```python
from build123d import *

# Parameters (mm, degrees)
SKETCH1_W                    = 44.45
SKETCH1_H                    = 12.7
SKETCH1_H_2                  = 15.875
SKETCH1_W_2                  = 41.275
BOSS_EXTRUDE1_DEPTH          = 3.175
SKETCH3_R                    = 14.2875
CUT_EXTRUDE1_DEPTH           = 68.351920908
F_18_0_1695_DIAMETER_HOLE1_D = 4.3053
CIRPATTERN1_COUNT            = 4
FILLET1_R                    = 6.35
FILLET2_R                    = 6.35
F_18_0_1695_DIAMETER_HOLE2_D = 4.3053


with BuildPart() as part:
    # Sketch1 → Boss-Extrude1 (new body)
    with BuildSketch(Plane(origin=(0, 0, 0), x_dir=(1, 0, 0), z_dir=(0, 1, 0))):
        Rectangle(SKETCH1_W, SKETCH1_H)
        with Locations((0, -14.2875)):
            Rectangle(SKETCH1_W, SKETCH1_H_2)
        with Locations((42.8625, 0)):
            Rectangle(SKETCH1_W_2, SKETCH1_H)
        with Locations((0, 14.2875)):
            Rectangle(SKETCH1_W, SKETCH1_H_2)
        with Locations((-42.8625, 0)):
            Rectangle(SKETCH1_W_2, SKETCH1_H)
    extrude(amount=BOSS_EXTRUDE1_DEPTH)

    # Sketch3 → Cut-Extrude1 (cut, through all)
    with BuildSketch(Plane(origin=(0, 3.175, 0), x_dir=(1, 0, 0), z_dir=(0, 1, 0))):
        with Locations(Location((0, 0, 0), (0, 0, 270))):
            Circle(SKETCH3_R)
    extrude(amount=-CUT_EXTRUDE1_DEPTH, mode=Mode.SUBTRACT)

    # #18 (0.1695) Diameter Hole1 (through all)
    with Locations(Plane(origin=(0, 3.175, 0), x_dir=(1, 0, 0), z_dir=(0, 1, 0))):
        with Locations((-15.715448212, -15.715448212)):
            f_18_0_1695_diameter_hole1 = Hole(F_18_0_1695_DIAMETER_HOLE1_D / 2)

    # CirPattern1: #18 (0.1695) Diameter Hole1 ×4 about axis
    cirpattern1_axis = Axis((0, 0, 0), (0, 1, 0))
    for i in range(1, CIRPATTERN1_COUNT):
        add(f_18_0_1695_diameter_hole1.rotate(cirpattern1_axis, i * 360 / CIRPATTERN1_COUNT), mode=Mode.SUBTRACT)

    # Fillet1
    fillet1_edges = [part.edges().sort_by_distance(p)[0] for p in [
        (-22.225, 1.5875, 6.35),
        (-22.225, 1.5875, -6.35),
        (22.225, 1.5875, -6.35),
        (22.225, 1.5875, 6.35),
    ]]
    fillet(fillet1_edges, radius=FILLET1_R)

    # Fillet2
    fillet2_edges = [part.edges().sort_by_distance(p)[0] for p in [
        (-63.5, 1.5875, 6.35),
        (-63.5, 1.5875, -6.35),
        (-22.225, 1.5875, -22.225),
        (22.225, 1.5875, -22.225),
        (63.5, 1.5875, -6.35),
        (63.5, 1.5875, 6.35),
        (22.225, 1.5875, 22.225),
        (-22.225, 1.5875, 22.225),
    ]]
    fillet(fillet2_edges, radius=FILLET2_R - 0.0001)  # a hair under: the kernel refuses the full size

    # #18 (0.1695) Diameter Hole2 (through all)
    with Locations(Plane(origin=(0, 3.175, 0), x_dir=(1, 0, 0), z_dir=(0, 1, 0))):
        with Locations((44.45, 0), (57.15, 0)):
            f_18_0_1695_diameter_hole2 = Hole(F_18_0_1695_DIAMETER_HOLE2_D / 2)

    # Mirror1: #18 (0.1695) Diameter Hole2 across plane
    add(f_18_0_1695_diameter_hole2.mirror(Plane(origin=(0, 0, 0), x_dir=(0, 0, 1), z_dir=(1, 0, 0))), mode=Mode.SUBTRACT)


solid = part.part
```
Input: part model. Units: mm. Frame: model coordinates. A direction names the side the tool comes from. Round coordinates to 2 decimals unless told otherwise and drop trailing zeros. Loops run counter-clockwise (first coordinate to the right, second up) from the corner with the lowest first, then second, coordinate; pieces in that order, holes last. Notation, with made-up numbers: M -30,55 L 27,55 A17 cw 27,75 Z; hole C -26.75,-35 d2. An arc over 180 degrees is marked long. Answer in a Markdown table with one row per item. Add a question column.
1. Section B-B (y = 0.85). Give the number of separate pieces and of enclosed holes in the cut face, and give its area (3 significant figures).
2. Contact query for flat-ended pins moving along their axis: pin 1 (4 mm diameter, centred on x = 15.72, z = 15.72, fed in from +Y); pin 2 (1.6 mm diameter, centred on x = -39.5, y = 1.5, fed in from -Z); pin 3 (1.6 mm diameter, centred on x = 39.5, y = 1, fed in from +Z). Output: stop coordinate, or through.
3. Mould query, pull axis X, two halves, no side actions, for faces 6 (the face through (0, 2, 22.225)), 7 (the face through (-17.77, 1.57, 15.07)), 8 (the face through (-24.036, 1.61, 8.26)). Classes: released by +X, released by -X, zero draft, split by the parting line, or undercut.
4. Section D-D (x = 33). Output: boundary loops of the cut face in (y, z) (3 decimals), and give its area (3 significant figures).
5. Section C-C (x = -44.45). Output: boundary loops of the cut face in (y, z) (3 decimals), and give its area (3 significant figures).
6. Section A-A (x = 0). Output: boundary loops of the cut face in (y, z) (1 decimal).
7. Set-up query: faces 1 (the face through (-43, 2, -6.35)), 2 (the face through (0, 2, -22.225)), 3 (the face through (17.704, 1.565, -16.54)), 4 (the face through (-43, 2, 6.35)), 5 (the face through (43, 2, -6.35)). Return all of +Z, -Z, +X, -X, +Y, -Y with unobstructed straight access to the full face (end or side cutting, diameter ignored); none if empty.
8. Ray query, probe 1 along Z at (x, y) = (16, 1.5); probe 2 along X at (y, z) = (0.6, -17). Return the intervals inside material, ascending.
Values follow:
| question | item | result |
|---|---|---|
| 1 | separate pieces | 1 |
| 1 | enclosed holes | 9 |
| 1 | area | 2,230 mm^2 |
| 2 | pin 1 | through |
| 2 | pin 2 | z = -6.35 |
| 2 | pin 3 | z = 6.35 |
| 3 | face 6 | zero draft |
| 3 | face 7 | undercut |
| 3 | face 8 | released by -X |
| 4 | outline | M 0,-6.35 L 3.175,-6.35 L 3.175,6.35 L 0,6.35 Z |
| 4 | area | 40.3 mm^2 |
| 5 | outline | M 0,-6.35 L 3.175,-6.35 L 3.175,-2.153 L 0,-2.153 Z; M 0,2.153 L 3.175,2.153 L 3.175,6.35 L 0,6.35 Z |
| 5 | area | 26.7 mm^2 |
| 6 | outline | M 0,-22.2 L 3.2,-22.2 L 3.2,-14.3 L 0,-14.3 Z; M 0,14.3 L 3.2,14.3 L 3.2,22.2 L 0,22.2 Z |
| 7 | face 1 | -Z, -X, +Y, -Y |
| 7 | face 2 | -Z, +X, -X, +Y, -Y |
| 7 | face 3 | +Y, -Y |
| 7 | face 4 | +Z, -X, +Y, -Y |
| 7 | face 5 | -Z, +X, +Y, -Y |
| 8 | probe 1 | -22.22 to -17.85, -13.58 to 13.58, 17.85 to 22.22 |
| 8 | probe 2 | -22.12 to -17.44, -13.99 to 13.99, 17.44 to 22.12 |
